Could you check a few things on this drawing? It's one solid part, dimensions in mm from its lowest x, y, z. Give positions to 0.01 mm unless a question says otherwise; leave off trailing zeros. Order: outer loops, then holes, each group sorted by start corner. A loop starts at its lowest first (then second) coordinate and runs counter-clockwise, first axis right, second up. Notation, with made-up numbers: (47, 53.5) -> (86, 53.5) arc R12 ccw to (86, 65.5) -> close; hole circle Ø6 at (39, -23). An arc over 180 degrees is marked (long way). Use one line per item in the form item = value. Start each with the question number.
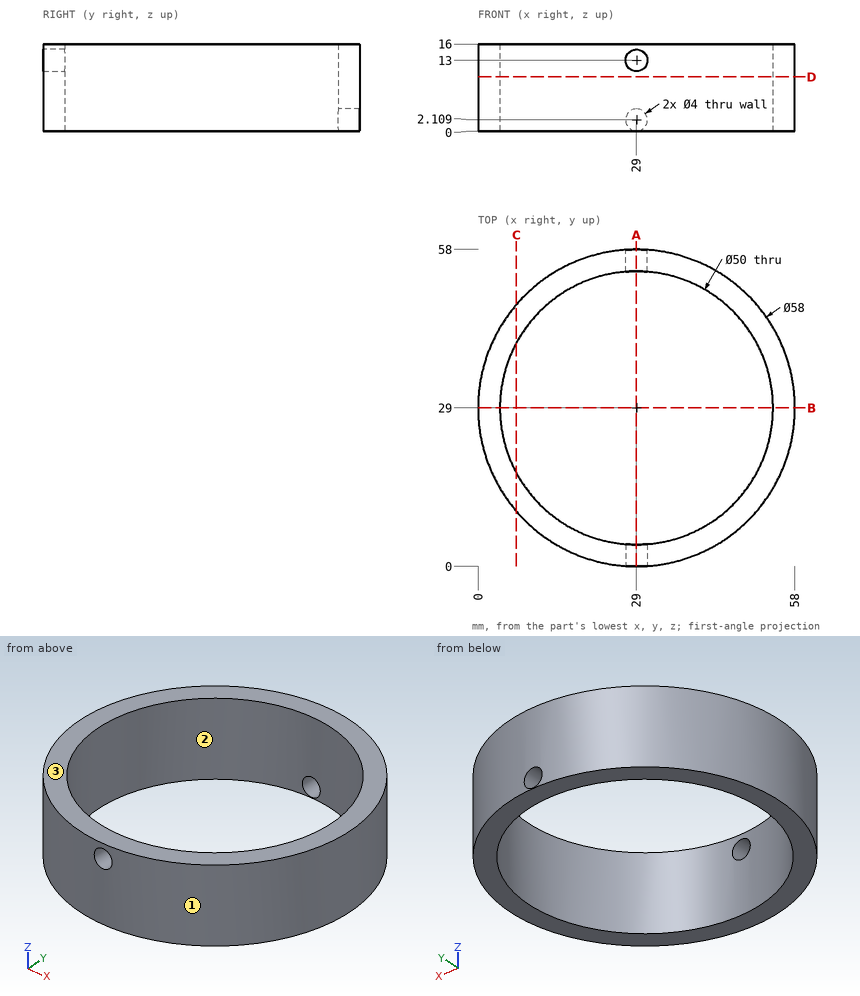
(1) Imagine slicing it at C-C (x = 7). Write out the boundary of the cut face in (y, z).
(2) We'd pull the mould along Y, two halves only. Please class the marked faces 1, 2 and 3: pulls with the +Y half, pulls with the -Y half, needs draft (parallel to the pull), parting line crosses it, or undercut.
(3) Imagine slicing it at D-D (z = 10). Write out the boundary of the cut face in (x, y), plus the area to 3 significant figures.
(4) Imagine slicing it at B-B (y = 29). Write out the boundary of the cut face in (x, z), plus the area to 3 significant figures.
(5) Imagine slicing it at A-A (x = 29). Write out the boundary of the cut face in (y, z).
(6) Please list where these lines run through material, in increasing order: probe 1 along Y at (x, z) = (29, 10); probe 2 along X at (y, z) = (3.5, 13); probe 3 along Y at (x, z) = (29.5, 1.75) (1 decimal).
(7) I'm going to push flat-ended pins straight in: pin 1 Ø3 at (y, z) = (7.5, 6) entering from -X; pin 2 Ø2 at (x, z) = (30.5, 14) entering from +Y; pin 3 Ø1 at (y, z) = (44, 3) entering from -X (1 decimal). Where does each tip first touch, or does it pass through?
Calculated:
q1.outline = (10.11, 0) -> (17.13, 0) -> (17.13, 16) -> (10.11, 16) -> close; (40.87, 0) -> (47.89, 0) -> (47.89, 16) -> (40.87, 16) -> close
q2.face_1 = parting line crosses it
q2.face_2 = undercut
q2.face_3 = needs draft
q3.outline = circle Ø58 at (29, 29); hole circle Ø50 at (29, 29)
q3.area = 679 mm2
q4.outline = (0, 0) -> (4, 0) -> (4, 16) -> (0, 16) -> close; (54, 0) -> (58, 0) -> (58, 16) -> (54, 16) -> close
q4.area = 128 mm2
q5.outline = (0, 0) -> (4, 0) -> (4, 11) -> (0, 11) -> close; (0, 15) -> (4, 15) -> (4, 16) -> (0, 16) -> close; (54, 0) -> (58, 0) -> (58, 0.11) -> (54, 0.11) -> close; (54, 4.11) -> (58, 4.11) -> (58, 16) -> (54, 16) -> close
q6.probe_1 = 0 to 4, 54 to 58
q6.probe_2 = 15.19 to 27, 31 to 42.81
q6.probe_3 = 0 to 4
q7.pin_1 = 8
q7.pin_2 = 58
q7.pin_3 = 3.9
